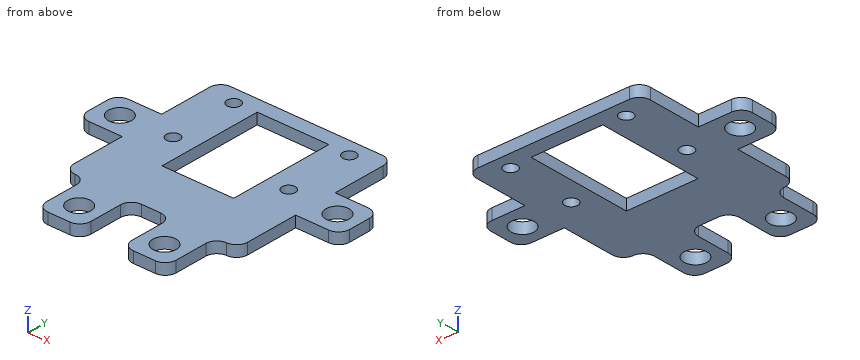
from build123d import *

# Parameters (mm, degrees)
SKETCH1_W             = 31.5
SKETCH1_H             = 31.5
SKETCH1_R             = 1.2
SKETCH1_W_2           = 13
SKETCH1_H_2           = 19.3
BOSS_EXTRUDE1_DEPTH   = 2
SKETCH4_W             = 8
SKETCH4_H             = 8
SKETCH4_R             = 2.1
BOSS_EXTRUDE3_DEPTH   = 2
CIRPATTERN2_OUTLINE_W = 8
CIRPATTERN2_OUTLINE_H = 8
CIRPATTERN2_OUTLINE_R = 2.1
CIRPATTERN2_DEPTH     = 2
SKETCH5_W             = 8
SKETCH5_H             = 10
SKETCH5_R             = 2.1
BOSS_EXTRUDE4_DEPTH   = 2
FILLET1_R             = 2


# Read off the part's stored shape, not the designer's step: CirPattern2
with BuildPart() as part:
    # Sketch1 → Boss-Extrude1 (new body)
    with BuildSketch(Plane.XY):
        with Locations((12.5, 9.25)):
            Rectangle(SKETCH1_W, SKETCH1_H)
        with Locations((2, 22)):
            Circle(SKETCH1_R, mode=Mode.SUBTRACT)
        with Locations((23, 22)):
            Circle(SKETCH1_R, mode=Mode.SUBTRACT)
        with Locations((23, 9.7)):
            Circle(SKETCH1_R, mode=Mode.SUBTRACT)
        with Locations((2, 9.7)):
            Circle(SKETCH1_R, mode=Mode.SUBTRACT)
        with Locations((12.5, 12.65)):
            Rectangle(SKETCH1_W_2, SKETCH1_H_2, mode=Mode.SUBTRACT)
    extrude(amount=BOSS_EXTRUDE1_DEPTH)

    # Sketch4 → Boss-Extrude3 (add)
    with BuildSketch(Plane.XY.offset(2)):
        with Locations((-7.25, 9.25)):
            Rectangle(SKETCH4_W, SKETCH4_H)
        with Locations((-7.25, 9.25)):
            Circle(SKETCH4_R, mode=Mode.SUBTRACT)
    extrude(amount=-BOSS_EXTRUDE3_DEPTH)

    # CirPattern2 outline → CirPattern2 (add)
    with BuildSketch(Plane.XY):
        with Locations((32.25, 9.25)):
            Rectangle(CIRPATTERN2_OUTLINE_W, CIRPATTERN2_OUTLINE_H)
        with Locations((32.25, 9.25)):
            Circle(CIRPATTERN2_OUTLINE_R, mode=Mode.SUBTRACT)
    extrude(amount=CIRPATTERN2_DEPTH)

    # Sketch5 → Boss-Extrude4 (add)
    # profile 1 of 2: a face of its own
    with BuildSketch(Plane(origin=(0, 0, 0), x_dir=(-1, 0, 0), z_dir=(0, 0, -1))):
        with Locations((-4.75, -11.5)):
            Rectangle(SKETCH5_W, SKETCH5_H)
        with Locations((-4.75, -12.4)):
            Circle(SKETCH5_R, mode=Mode.SUBTRACT)
    # profile 2 of 2: a face of its own
    with BuildSketch(Plane(origin=(0, 0, 0), x_dir=(-1, 0, 0), z_dir=(0, 0, -1))):
        with Locations((-20.25, -11.5)):
            Rectangle(SKETCH5_W, SKETCH5_H)
        with Locations(Location((-20.25, -12.4, 0), (0, 0, 180))):
            Circle(SKETCH5_R, mode=Mode.SUBTRACT)
    extrude(amount=-BOSS_EXTRUDE4_DEPTH)

    # Fillet1
    fillet1_edges = [part.edges().sort_by_distance(p)[0] for p in [
        (-11.25, 13.25, 1),
        (-11.25, 5.25, 1),
        (36.25, 5.25, 1),
        (36.25, 13.25, 1),
        (0.75, -6.5, 1),
        (0.75, -16.5, 1),
        (8.75, -16.5, 1),
        (8.75, -6.5, 1),
        (-3.25, 25, 1),
        (28.25, 25, 1),
        (28.25, -6.5, 1),
        (-3.25, -6.5, 1),
        (24.25, -16.5, 1),
        (24.25, -6.5, 1),
        (16.25, -6.5, 1),
        (16.25, -16.5, 1),
    ]]
    fillet(fillet1_edges, radius=FILLET1_R - 0.0001)  # a hair under: the kernel refuses the full size


solid = part.part
CAD build for the part. Positions are in the model's coordinates, mm. Round coordinates to 2 decimals unless told otherwise and drop trailing zeros. Order: outer loops, then holes, each group sorted by start corner. A loop starts at its lowest first (then second) coordinate and runs counter-clockwise, first axis right, second up. Notation, with made-up numbers: (69.5, 73) -> (78.5, 73) arc R19 ccw to (78.5, 91) -> close; hole circle Ø6 at (-19, 6). An arc over 180 degrees is marked (long way). Write item = value, one per line. Start each with the question number.
(1) Cut at C-C, the plane x = 2. List the corners of the cut face in (y, z).
(2) Cut at A-A, the plane y = -12.4. List the corners of the cut face in (x, z), then the cut area to 3 significant figures.
(3) Pin check, flat tips, straight feed: P1, Ø1, axis at x = 13.5, z = 1, coming from the -Y side; P2, Ø2.5, axis at x = -7.25, y = 9.25, coming from the -Z side; P3, Ø1, axis at y = -11, z = 1.5, coming from the +X side; P4, Ø1, axis at x = -7.5, z = 1, coming from the +Y side. Stop position of each tip, or through.
(4) Cut at D-D, the plane z = 0.9. State how many separate pieces and enclosed holes the cut face has, then the cut area to 3 significant figures.
(5) Probe line 1 (X direction, y = 20.5, z = 1.2); line 2 (Y direction, x = 23, z = 0.95); line 3 (Y direction, x = -7.25, z = 0.7). List the from-to ranges inside material, lowest first. Write a range as [from, to].
(6) Cut at B-B, the plane x = 20.25. List the corners of the cut face in (y, z).
Model answer:
q1.outline = (-16.35, 0) -> (8.5, 0) -> (8.5, 2) -> (-16.35, 2) -> close; (10.9, 0) -> (20.8, 0) -> (20.8, 2) -> (10.9, 2) -> close; (23.2, 0) -> (25, 0) -> (25, 2) -> (23.2, 2) -> close
q2.outline = (0.75, 0) -> (2.65, 0) -> (2.65, 2) -> (0.75, 2) -> close; (6.85, 0) -> (8.75, 0) -> (8.75, 2) -> (6.85, 2) -> close; (16.25, 0) -> (18.15, 0) -> (18.15, 2) -> (16.25, 2) -> close; (22.35, 0) -> (24.25, 0) -> (24.25, 2) -> (22.35, 2) -> close
q2.area = 15.2 mm2
q3.P1 = -6.5
q3.P2 = through
q3.P3 = 24.25
q3.P4 = 13.25
q4.separate_pieces = 1
q4.enclosed_holes = 9
q4.area = 949 mm2
q5.line_1 = [-3.25, 6], [19, 28.25]
q5.line_2 = [-16.35, 8.5], [10.9, 20.8], [23.2, 25]
q5.line_3 = [5.25, 7.15], [11.35, 13.25]
q6.outline = (-16.5, 0) -> (-14.5, 0) -> (-14.5, 2) -> (-16.5, 2) -> close; (-10.3, 0) -> (25, 0) -> (25, 2) -> (-10.3, 2) -> close
